Here's how the part is built. I have some questions about the finished solid (model axes, mm). A direction names the side the tool comes from. Give positions to 0.01 mm unless a question says otherwise; leave off trailing zeros. Order: outer loops, then holes, each group sorted by start corner. A loop starts at its lowest first (then second) coordinate and runs counter-clockwise, first axis right, second up. Notation, with made-up numbers: (69, -1.75) - (119, -1.75) arc R37 ccw to (119, 34.25) - close; hole circle Ø9 at (81, 59). An arc over 180 degrees is marked (long way). One line per question, with ' | ' between items.
from build123d import *

# Parameters (mm, degrees)
COVER_BODY_DEPTH                        = 117
CBORE_FOR_M6_HEX_HEAD_BOLT1_D           = 6
CBORE_FOR_M6_HEX_HEAD_BOLT1_CBORE_D     = 12
CBORE_FOR_M6_HEX_HEAD_BOLT1_CBORE_DEPTH = 3
CBORE_FOR_M6_HEX_HEAD_BOLT2_D           = 6
CBORE_FOR_M6_HEX_HEAD_BOLT2_CBORE_D     = 12
CBORE_FOR_M6_HEX_HEAD_BOLT2_CBORE_DEPTH = 3
FILLET1_R                               = 5


with BuildPart() as part:
    # Sketch1 → Cover Body (new body)
    with BuildSketch(Plane.XY):
        Polygon((-17.507754177, -4.568983292), (16.992245823, 11.631016708), (37.567245823, 11.631016708), (37.567245823, 6.631016708), (16.992245823, 6.631016708), (-17.507754177, -9.568983292), (-38.082754177, -9.568983292), (-38.082754177, -4.568983292), align=None)
    extrude(amount=-COVER_BODY_DEPTH)

    # CBORE for M6 Hex Head Bolt1 (through all)
    with Locations(Plane(origin=(0, -4.568983292, 0), x_dir=(1, 0, 0), z_dir=(0, 1, 0))):
        with Locations((-30.582754177, 109.5), (-30.582754177, 7.5)):
            CounterBoreHole(CBORE_FOR_M6_HEX_HEAD_BOLT1_D / 2, CBORE_FOR_M6_HEX_HEAD_BOLT1_CBORE_D / 2, CBORE_FOR_M6_HEX_HEAD_BOLT1_CBORE_DEPTH)

    # CBORE for M6 Hex Head Bolt2 (through all)
    with Locations(Plane(origin=(0, 11.631016708, 0), x_dir=(1, 0, 0), z_dir=(0, 1, 0))):
        with Locations((30.067245823, 7.5), (30.067245823, 109.5)):
            CounterBoreHole(CBORE_FOR_M6_HEX_HEAD_BOLT2_D / 2, CBORE_FOR_M6_HEX_HEAD_BOLT2_CBORE_D / 2, CBORE_FOR_M6_HEX_HEAD_BOLT2_CBORE_DEPTH)

    # Fillet1
    fillet1_edges = [part.edges().sort_by_distance(p)[0] for p in [
        (37.567245823, 9.131016708, 0),
        (37.567245823, 9.131016708, -117),
        (-38.082754177, -7.068983292, -117),
        (-38.082754177, -7.068983292, 0),
    ]]
    fillet(fillet1_edges, radius=FILLET1_R)


solid = part.part
1) I want a section at A-A (z = -109.5). List the corners of the cut face in (x, y) for me, plus the area to 3 significant figures.
Model answer:
outline: (-38.08, -9.57) - (-33.58, -9.57) - (-33.58, -7.57) - (-36.58, -7.57) - (-36.58, -4.57) - (-38.08, -4.57) - close; (-27.58, -9.57) - (-17.51, -9.57) - (16.99, 6.63) - (27.07, 6.63) - (27.07, 8.63) - (24.07, 8.63) - (24.07, 11.63) - (16.99, 11.63) - (-17.51, -4.57) - (-24.58, -4.57) - (-24.58, -7.57) - (-27.58, -7.57) - close; (33.07, 6.63) - (37.57, 6.63) - (37.57, 11.63) - (36.07, 11.63) - (36.07, 8.63) - (33.07, 8.63) - close | area: 282 mm2
2) I want a section at D-D (x = 12). List the corners of the cut face in (y, z) for me, plus the area to 3 significant figures.
Model answer:
outline: (4.29, -117) - (9.29, -117) - (9.29, 0) - (4.29, 0) - close | area: 585 mm2
3) Please list where these lines run through material, in increasing order: L1, parallel to Y at x = 18, z = -24.5; L2, parallel to Y at x = -34, z = -108; L3, parallel to X at y = 1.25, z = -10.
Model answer:
L1: y = 6.63 to 11.63 | L2: y = -9.57 to -7.57 | L3: x = -5.12 to 5.53
4) Thinking about a two-plate mould opening in X: for faces 1 (the face through (-0.016, -1.356, -57.681)), 2 (the face through (27, 11.631, -58)), 3 (the face through (33.29, 10.15, -114.56)), which applies, +X half, -X half, draft (parallel to the pull), parting line (faces both ways), or undercut?
Model answer:
face 1: +X half | face 2: draft | face 3: undercut
5) On a 3-axis mill with a long thin cutter (end or side, diameter ignored), from which of +Z, -Z, +X, -X, +Y, -Y can I reach the whole of each face in a straight line? I mean faces 4 (the face through (27, 6.631, -58)), 5 (the face through (37.567, 9, -58)), 6 (the face through (-28, -7.569, -107)). Say none if no direction works.
Model answer:
face 4: +Z, -Z, +X, -Y | face 5: +Z, -Z, +X, +Y, -Y | face 6: +Y
6) I want a section at B-B (z = -69.5). List the corners of the cut face in (x, y) for me.
Model answer:
outline: (-38.08, -9.57) - (-17.51, -9.57) - (16.99, 6.63) - (37.57, 6.63) - (37.57, 11.63) - (16.99, 11.63) - (-17.51, -4.57) - (-38.08, -4.57) - close
7) I'm going to push flat-ended pins straight in: P1, Ø4, axis at x = -2, z = -103.5, coming from the +Y side; P2, Ø6, axis at x = -31.5, z = -8, coming from the +Y side; P3, Ø1.5, axis at x = -27, z = -27, coming from the +Y side; P4, Ø3.5, axis at x = 30.07, z = -109.5, coming from the -Y side. Where does each tip first touch, or does it pass through?
Model answer:
P1: stops at y = 3.65 | P2: stops at y = -7.57 | P3: stops at y = -4.57 | P4: passes through
8) I want a section at C-C (y = -6). List the corners of the cut face in (x, z) for me.
Model answer:
outline: (-38.08, -112) arc R5 ccw to (-33.08, -117) - (-9.91, -117) - (-9.91, 0) - (-33.08, 0) arc R5 ccw to (-38.08, -5) - close; hole circle Ø12 at (-30.58, -109.5); hole circle Ø12 at (-30.58, -7.5)
